from build123d import *

# Parameters (mm, degrees)
SKETCH1_R            = 50.800375113
SKETCH1_R_2          = 47.812951641
BOSS_EXTRUDE2_DEPTH  = 350
BOSS_EXTRUDE5_DEPTH  = 50
BOSS_EXTRUDE11_DEPTH = 50
SKETCH6_R            = 44.996318031
CUT_EXTRUDE2_DEPTH   = 50
SKETCH7_R            = 43.517898498
CUT_EXTRUDE3_DEPTH   = 50
SKETCH10_W           = 19.115808835
SKETCH10_H           = 20.742352913
BOSS_EXTRUDE12_DEPTH = 50
SKETCH11_W           = 54.364903868
SKETCH11_H           = 26.370020035
CUT_EXTRUDE6_DEPTH   = 50
SKETCH12_W           = 154.555587183
SKETCH12_H           = 189.686795077
CUT_EXTRUDE7_DEPTH   = 434.835259258
CUT_EXTRUDE9_DEPTH   = 50


with BuildPart() as part:
    # Sketch1 → Boss-Extrude2 (new body)
    with BuildSketch(Plane(origin=(0, 0, 0), x_dir=(0, 0, -1), z_dir=(1, 0, 0))):
        with Locations((1.289702318, 0)):
            Circle(SKETCH1_R)
        with Locations((1.289702318, 0)):
            Circle(SKETCH1_R_2, mode=Mode.SUBTRACT)
    extrude(amount=BOSS_EXTRUDE2_DEPTH)

    # Sketch3 → Boss-Extrude5 (add)
    with BuildSketch(Plane(origin=(350, 0, 0), x_dir=(0, 0, -1), z_dir=(1, 0, 0))):
        Polygon((58.055626726, -36.855405481), (60.945530776, 31.849944836), (2.88990405, 68.705350317), (-58.055626726, 36.855405481), (-60.945530776, -31.849944836), (-2.88990405, -68.705350317), align=None)
        Polygon((29.411876605, -18.99044871), (30.315925302, 11.383738416), (4.46313198, 27.353761118), (-22.293710039, 12.949596693), (-23.197758737, -17.424590433), (2.655034585, -33.394613135), align=None, mode=Mode.SUBTRACT)
    extrude(amount=BOSS_EXTRUDE5_DEPTH)

    # Sketch5 → Boss-Extrude11 (add)
    with BuildSketch(Plane.ZY):
        Polygon((0, -67.161353017), (58.163437865, -33.580676508), (58.163437865, 33.580676508), (0, 67.161353017), (-58.163437865, 33.580676508), (-58.163437865, -33.580676508), align=None)
    extrude(amount=BOSS_EXTRUDE11_DEPTH)

    # Sketch6 → Cut-Extrude2 (cut)
    with BuildSketch(Plane(origin=(0, 0, 0), x_dir=(0, 0, -1), z_dir=(1, 0, 0))):
        with Locations((2.167278034, 0)):
            Circle(SKETCH6_R)
    extrude(amount=-CUT_EXTRUDE2_DEPTH, mode=Mode.SUBTRACT)

    # Sketch7 → Cut-Extrude3 (cut)
    with BuildSketch(Plane.ZY.offset(-350)):
        with Locations((-2.231478452, -1.09442532)):
            Circle(SKETCH7_R)
    extrude(amount=-CUT_EXTRUDE3_DEPTH, mode=Mode.SUBTRACT)

    # Sketch10 → Boss-Extrude12 (add)
    with BuildSketch(Plane(origin=(0, 50.277647577, -31.917717413), x_dir=(1, 0, 0), z_dir=(0, 0.8442477544511112, -0.5359531034561291))):
        with Locations((368.704344308, -19.961055073)):
            Rectangle(SKETCH10_W, SKETCH10_H)
    extrude(amount=BOSS_EXTRUDE12_DEPTH)

    # Sketch11 → Cut-Extrude6 (cut)
    with BuildSketch(Plane(origin=(378.262248725, 0, 0), x_dir=(0, 0, -1), z_dir=(1, 0, 0))):
        with Locations((35.769872333, 101.000183765)):
            Rectangle(SKETCH11_W, SKETCH11_H)
    extrude(amount=-CUT_EXTRUDE6_DEPTH, mode=Mode.SUBTRACT)

    # Sketch12 → Cut-Extrude7 (cut, through all)
    with BuildSketch(Plane(origin=(0, 87.815173747, 0), x_dir=(1, 0, 0), z_dir=(0, 1, 0))):
        with Locations((171.244586456, 101.756488253)):
            Rectangle(SKETCH12_W, SKETCH12_H)
    extrude(amount=-CUT_EXTRUDE7_DEPTH, mode=Mode.SUBTRACT)

    # Sketch13 → Cut-Extrude9 (cut)
    with BuildSketch(Plane(origin=(378.262248725, 0, 0), x_dir=(0, 0, -1), z_dir=(1, 0, 0))):
        Polygon((2.767415971, 94.353770173), (53.126909072, 94.353770173), (23.904702859, 55.316039855), (1.784436984, 69.406798444), align=None)
    extrude(amount=-CUT_EXTRUDE9_DEPTH, mode=Mode.SUBTRACT)


solid = part.part
Source: CAD feature listing. Evaluate the final solid. Frame: model axes, mm. A direction names the side the tool comes from. Give positions to 0.01 mm unless a question says otherwise; leave off trailing zeros. Write each loop counter-clockwise with the first axis right and the second up, starting at its lowest first coordinate (ties: lowest second). Pieces come first, ordered by that corner, then holes. Notation, with made-up numbers: M 82,0 L 90,0 A21 ccw 90,16 Z; hole C 57.5,-40 d4. An arc over 180 degrees is marked long. Return JSON: item names as keys, results as strings. Group by question number.
1) Cut plane D-D, the plane x = 258.5. Output: boundary loops of the cut face in (y, z), plus the area to 3 significant figures.
2) Material intervals for line 1 along X through (y, z) = (38.5, -32.5); line 2 along X through (y, z) = (49, 24); line 3 along Y through (x, z) = (373.5, 17.5), sorted ascending. Write a range as [from, to].
3) Pull-direction query (X, two-part tool) for faces 1 (the face through (0, -49, 13)), 2 (the face through (93.967, 0.2, -49.5)), 3 (the face through (-24.65, 30.41, 31)), 4 (the face through (400, 1, 41.5)); classes: pulls with the +X half, pulls with the -X half, needs draft (parallel to the pull), parting line crosses it, or undercut.
4) Set-up query: faces 5 (the face through (172.55, 2.102, 46.477)), 6 (the face through (-25, 0, -58.163)), 7 (the face through (-24.65, 50.61, -28.67)). Return all of +Z, -Z, +X, -X, +Y, -Y with unobstructed straight access to the full face (end or side cutting, diameter ignored); none if empty.
5) Cut plane B-B, the plane z = 33. Output: boundary loops of the cut face in (x, y).
6) Cut plane C-C, the plane y = 60.5. Output: boundary loops of the cut face in (x, z), plus the area to 3 significant figures.
7) Pin query (flat end, axial travel): P1, Ø3, axis at x = 132, z = 35.5, coming from the -Y side; P2, Ø25, axis at x = -30.5, y = 9, coming from the -Z side; P3, Ø1.5, axis at x = 164.5, y = -48.5, coming from the -Z side. Return the tip coordinate at first contact, or that it passes through.
8) Cut plane A-A, the plane y = 22.5. Output: boundary loops of the cut face in (x, z), plus the area to 3 significant figures.
Recorded:
{
 "1": {"outline": "C 0,-1.29 d101.6; hole C 0,-1.29 d95.63", "area": "926 mm²"},
 "2": {"line 1": "x = [-50, 93.97], [248.52, 400]", "line 2": "x = [-50, 0], [350, 400]", "line 3": "y = [-59.43, -39.88], [37.69, 58.05]"},
 "3": {"face 1": "undercut", "face 2": "undercut", "face 3": "needs draft", "face 4": "pulls with the +X half"},
 "4": {"face 5": "none", "face 6": "-Z, -X, +Y, -Y", "face 7": "-Z, -X, +Y"},
 "5": {"outline": "M -50,-48.11 L 0,-48.11 L 0,-37.48 L 350,-37.48 L 350,-49.59 L 400,-49.59 L 400,-26.64 L 350,-26.64 L 350,-33.32 L 0,-33.32 L 0,-28.07 L -50,-28.07 Z; M -50,28.07 L 0,28.07 L 0,33.32 L 350,33.32 L 350,24.45 L 400,24.45 L 400,49.95 L 350,49.95 L 350,37.48 L 0,37.48 L 0,48.11 L -50,48.11 Z"},
 "6": {"outline": "M -50,-11.54 L 0,-11.54 L 0,11.54 L -50,11.54 Z; M 350,-15.77 L 378.26,-15.77 L 378.26,-15.82 L 400,-15.82 L 400,12.81 L 350,12.81 Z", "area": "2,580 mm²"},
 "7": {"P1": "stops at y = -36.54", "P2": "stops at z = -58.16", "P3": "stops at z = -6.91"},
 "8": {"outline": "M -50,-58.16 L 0,-58.16 L 0,-46.84 L 93.97,-46.84 L 93.97,-43.48 L 0,-43.48 L 0,-41.13 L -50,-41.13 Z; M -50,36.8 L 0,36.8 L 0,40.9 L 350,40.9 L 350,34.34 L 400,34.34 L 400,58.66 L 350,58.66 L 350,44.26 L 0,44.26 L 0,58.16 L -50,58.16 Z; M 248.52,-46.84 L 350,-46.84 L 350,-60.55 L 400,-60.55 L 400,-38.8 L 350,-38.8 L 350,-43.48 L 248.52,-43.48 Z", "area": "6,060 mm²"}
}
